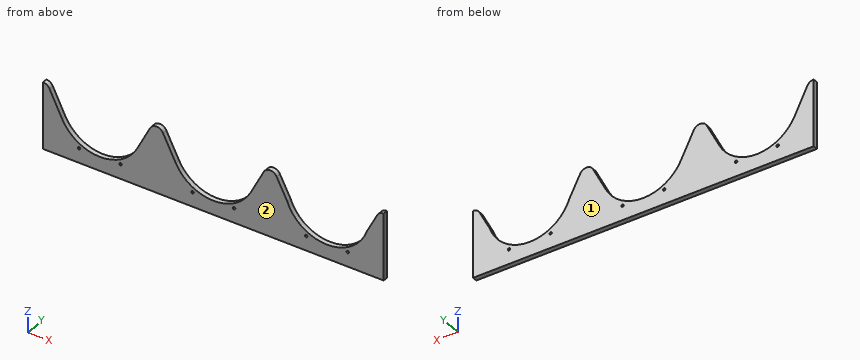
from build123d import *

# Parameters (mm, degrees)
SKETCH1_R           = 1.6383
BOSS_EXTRUDE1_DEPTH = 6.35
FILLET3_R           = 9.525


with BuildPart() as part:
    # Sketch1 → Boss-Extrude1 (new body)
    with BuildSketch(Plane(origin=(0, 0, 0), x_dir=(1, 0, 0), z_dir=(0, 1, 0))):
        with BuildLine():
            Line((-155.195517325, 13.78007871), (-129.789904869, -35.823423436))
            Line((-129.789904869, -35.823423436), (-104.384292413, 13.78007871))
            ThreePointArc((-104.384292413, 13.78007871), (-54.648238202, 44.186576564), (-4.912183992, 13.78007871))
            Line((-4.912183992, 13.78007871), (20.493428464, -35.823423436))
            Line((20.493428464, -35.823423436), (43.089138197, 7.319646013))
            ThreePointArc((43.089138197, 7.319646013), (95.947099994, 44.185705521), (148.390090675, 6.731691085))
            Line((148.390090675, 6.731691085), (162.314428993, -20.219790589))
            ThreePointArc((162.314428993, -20.219790589), (165.822867077, -23.983160647), (170.776761798, -25.372771775))
            Line((170.776761798, -25.372771775), (170.776761798, 62.601576564))
            Line((170.776761798, 62.601576564), (-280.073238202, 62.601576564))
            Line((-280.073238202, 62.601576564), (-280.073238202, -25.107798436))
            ThreePointArc((-280.073238202, -25.107798436), (-275.072672567, -23.689583762), (-271.561214661, -19.857266851))
            Line((-271.561214661, -19.857266851), (-254.868776311, 13.383457934))
            ThreePointArc((-254.868776311, 13.383457934), (-205.153928001, 44.186134164), (-155.195517325, 13.78007871))
        make_face()
        with Locations(Location((-232.439771536, 43.551576564, 0), (0, 0, 270))):
            Circle(SKETCH1_R, mode=Mode.SUBTRACT)
        with Locations(Location((-177.423371536, 43.551576564, 0), (0, 0, 270))):
            Circle(SKETCH1_R, mode=Mode.SUBTRACT)
        with Locations(Location((-27.140038202, 43.551576564, 0), (0, 0, 270))):
            Circle(SKETCH1_R, mode=Mode.SUBTRACT)
        with Locations(Location((-82.156438202, 43.551576564, 0), (0, 0, 270))):
            Circle(SKETCH1_R, mode=Mode.SUBTRACT)
        with Locations(Location((123.143295131, 43.551576564, 0), (0, 0, 270))):
            Circle(SKETCH1_R, mode=Mode.SUBTRACT)
        with Locations(Location((68.126895131, 43.551576564, 0), (0, 0, 270))):
            Circle(SKETCH1_R, mode=Mode.SUBTRACT)
    extrude(amount=-BOSS_EXTRUDE1_DEPTH)

    # Fillet3
    fillet3_edges = [part.edges().sort_by_distance(p)[0] for p in [
        (20.493428464, -3.175, 35.823423436),
        (-129.789904869, -3.175, 35.823423436),
    ]]
    fillet(fillet3_edges, radius=FILLET3_R)


solid = part.part
Read the model definition and answer for the solid it produces. Units are mm, in the model's axes. Face numbers are marked on the shaded views. Round coordinates to 2 decimals unless told otherwise and drop trailing zeros. Order: outer loops, then holes, each group sorted by start corner. A loop starts at its lowest first (then second) coordinate and runs counter-clockwise, first axis right, second up.
1) The part is cut by section B-B on y = -4.75. Write down the section's boundary in (x, z) (3 decimals).
2) The part is cut by section C-C on x = -21. Write down the section's boundary in (y, z), plus the area to 3 significant figures.
3) The part is cut by section A-A on z = 15.5. Write down the section's boundary in (x, y), plus the area to 3 significant figures.
4) The mould has two halves that part along Y. Classify the marked faces 1 and 2: released by +Y, released by -Y, zero draft, split by the parting line, or undercut.
5) The part is cut by section D-D on x = -248. Write down the section's boundary in (y, z), plus the area to 3 significant figures.
6) Straight lines are drawn through the part: L1, parallel to X at y = -0.25, z = -39.5; L2, parallel to X at y = -5.5, z = -21; L3, parallel to Z at x = -55, y = -0.25. For each, find the intervals that lie inside material, in ascending order.
7) Flat-ended cylindrical pins translate along their axes: pin 1 (2 mm diameter, centred on x = -232.44, z = -43.55, fed in from +Y); pin 2 (2 mm diameter, centred on x = -124, y = -1, fed in from +Z). Find the tip coordinate at first contact, or state that the pin passes through.
Resolved:
1. outline: (-280.073, -62.602) - (170.777, -62.602) - (170.777, 25.373) arc R9.525 ccw to (162.314, 20.22) - (148.39, -6.732) arc R55.88 cw to (43.089, -7.32) - (29.026, 19.532) arc R9.525 ccw to (12.11, 19.455) - (-4.912, -13.78) arc R55.88 cw to (-104.384, -13.78) - (-121.312, 19.271) arc R9.525 ccw to (-138.268, 19.271) - (-155.196, -13.78) arc R55.88 cw to (-254.869, -13.383) - (-271.561, 19.857) arc R9.525 ccw to (-280.073, 25.108) - close; hole circle Ø3.277 at (-232.44, -43.552); hole circle Ø3.277 at (-177.423, -43.552); hole circle Ø3.277 at (-82.156, -43.552); hole circle Ø3.277 at (-27.14, -43.552); hole circle Ø3.277 at (68.127, -43.552); hole circle Ø3.277 at (123.143, -43.552)
2. outline: (-6.35, -62.6) - (0, -62.6) - (0, -32.92) - (-6.35, -32.92) - close
2. area: 188 mm2
3. outline: (-280.07, -6.35) - (-269.37, -6.35) - (-269.37, 0) - (-280.07, 0) - close; (-140.2, -6.35) - (-119.38, -6.35) - (-119.38, 0) - (-140.2, 0) - close; (10.08, -6.35) - (31.14, -6.35) - (31.14, 0) - (10.08, 0) - close; (159.88, -6.35) - (170.78, -6.35) - (170.78, 0) - (159.88, 0) - close
3. area: 403 mm2
4. face 1: released by +Y
4. face 2: released by -Y
5. outline: (-6.35, -62.6) - (0, -62.6) - (0, -23.91) - (-6.35, -23.91) - close
5. area: 246 mm2
6. L1: x = -280.07 to -227.33, -182.53 to -77.05, -32.25 to 73.23, 118.04 to 170.78
6. L2: x = -280.07 to -250.25, -159.61 to -99.97, -9.33 to 50.32, 140.95 to 170.78
6. L3: z = -62.6 to -44.19
7. pin 1: passes through
7. pin 2: stops at z = 23.16
